Model file for the job. Use its own axes, mm. Face numbers are marked on the shaded views. A direction names the side the tool comes from. Coordinates: 2 decimals unless noted, no trailing zeros. Write each loop counter-clockwise with the first axis right and the second up, starting at its lowest first coordinate (ties: lowest second). Pieces come first, ordered by that corner, then holes. Notation, with made-up numbers: (13, -18.5) - (26, -18.5) arc R9 cw to (26, -1.5) - close; hole circle Ø4 at (0, 30.25). An arc over 180 degrees is marked (long way). Put each result on its own line as item: value. Start each with the question number.
1. Saw through at D-D, the plane z = 46. Write the cut outline in (x, y).
2. Drill centre lines: L1, parallel to X at y = 24.2, z = 46; L2, parallel to Z at x = 15.5, y = 24.05; L3, parallel to Z at x = 0, y = 23. Where is each one in solid material? Low to high. Write a range as from..to.
3. Which spindle directions (+Z, -Z, +X, -X, +Y, -Y) get a long thin tool onto all of the face, cutting with end or side? Do the marked faces 1 and 2. Say none if no direction does.
4. Saw through at A-A, the plane z = 30. Write the cut outline in (x, y), plus the area to 3 significant figures.
5. Saw through at B-B, the plane y = -9.5. Write the cut outline in (x, z).
6. Saw through at C-C, the plane x = 0. Write the cut outline in (y, z).
7. Drop flat-ended pins along their axis: P1, Ø1.5, axis at x = -3.5, y = -3.5, coming from the -Z side; P2, Ø14.5, axis at x = 12, z = 25, coming from the -Y side; P3, Ø6, axis at y = 17.5, z = 8.5, coming from the +X side (3 decimals); P4, Ø14.5, axis at x = -8, y = -12, coming from the +Z side. Give the stop position or say it passes through.
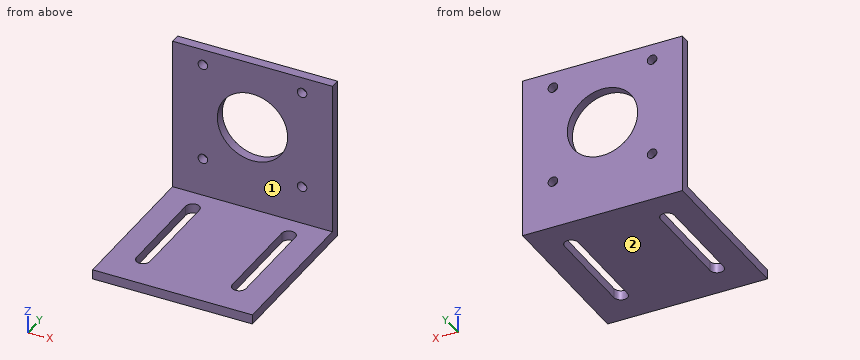
```python
from build123d import *

# Parameters (mm, degrees)
SKETCH1_W               = 50
SKETCH1_H               = 51
BOSS_EXTRUDE1_DEPTH     = 3
SKETCH2_W               = 50
SKETCH2_H               = 3
BOSS_EXTRUDE2_DEPTH     = 48
CUT_EXTRUDE1_DEPTH      = 75.36396977
CUT_EXTRUDE1_DEPTH_BACK = 75.36396977
SKETCH3_R               = 11
SKETCH3_R_2             = 1.5


with BuildPart() as part:
    # Sketch1 → Boss-Extrude1 (new body)
    with BuildSketch(Plane.XY):
        Rectangle(SKETCH1_W, SKETCH1_H)
        with BuildLine():
            Line((-17.15, 15.35), (-17.15, -14.35))
            ThreePointArc((-17.15, -14.35), (-15, -16.5), (-12.85, -14.35))
            Line((-12.85, -14.35), (-12.85, 15.35))
            ThreePointArc((-12.85, 15.35), (-15, 17.5), (-17.15, 15.35))
        make_face(mode=Mode.SUBTRACT)
        with BuildLine():
            Line((12.88, 15.35), (12.88, -14.35))
            ThreePointArc((12.88, -14.35), (15.03, -16.5), (17.18, -14.35))
            Line((17.18, -14.35), (17.18, 15.35))
            ThreePointArc((17.18, 15.35), (15.03, 17.5), (12.88, 15.35))
        make_face(mode=Mode.SUBTRACT)
    extrude(amount=BOSS_EXTRUDE1_DEPTH)

    # Sketch2 → Boss-Extrude2 (add)
    with BuildSketch(Plane.XY.offset(3)):
        with Locations((0, 24)):
            Rectangle(SKETCH2_W, SKETCH2_H)
    extrude(amount=BOSS_EXTRUDE2_DEPTH)

    # Sketch3 → Cut-Extrude1 (cut, two sides: drawn at the far end of the back side and taken through both)
    with BuildSketch(Plane.XZ.offset(-22.5).offset(-CUT_EXTRUDE1_DEPTH_BACK)):
        with Locations((0, 30)):
            Circle(SKETCH3_R)
        with Locations((-15.5, 46)):
            Circle(SKETCH3_R_2)
        with Locations((15.5, 46)):
            Circle(SKETCH3_R_2)
        with Locations((-15.5, 15)):
            Circle(SKETCH3_R_2)
        with Locations((15.5, 15)):
            Circle(SKETCH3_R_2)
    extrude(amount=CUT_EXTRUDE1_DEPTH + CUT_EXTRUDE1_DEPTH_BACK, mode=Mode.SUBTRACT)


solid = part.part
```
Final values:
1. outline: (-25, 22.5) - (-17, 22.5) - (-17, 25.5) - (-25, 25.5) - close; (-14, 22.5) - (14, 22.5) - (14, 25.5) - (-14, 25.5) - close; (17, 22.5) - (25, 22.5) - (25, 25.5) - (17, 25.5) - close
2. L1: x = -25..-17, -14..14, 17..25
2. L2: z = 0..13.5, 16.5..44.5, 47.5..51
2. L3: z = 0..19, 41..51
3. face 1: +Z, +X, -X, -Y
3. face 2: -Z, +X, -X, +Y, -Y
4. outline: (-25, 22.5) - (-11, 22.5) - (-11, 25.5) - (-25, 25.5) - close; (11, 22.5) - (25, 22.5) - (25, 25.5) - (11, 25.5) - close
4. area: 84.0 mm²
5. outline: (-25, 0) - (-17.15, 0) - (-17.15, 3) - (-25, 3) - close; (-12.85, 0) - (12.88, 0) - (12.88, 3) - (-12.85, 3) - close; (17.18, 0) - (25, 0) - (25, 3) - (17.18, 3) - close
6. outline: (-25.5, 0) - (25.5, 0) - (25.5, 19) - (22.5, 19) - (22.5, 3) - (-25.5, 3) - close; (22.5, 41) - (25.5, 41) - (25.5, 51) - (22.5, 51) - close
7. P1: stops at z = 0
7. P2: stops at y = 22.5
7. P3: passes through
7. P4: stops at z = 3
